Here's how the part is built. I have some questions about the finished solid (model axes, mm). Round coordinates to 2 decimals unless told otherwise and drop trailing zeros. Loops run counter-clockwise (first coordinate to the right, second up) from the corner with the lowest first, then second, coordinate; pieces in that order, holes last. Notation, with made-up numbers: M -11,57.25 L 37,57.25 A8 ccw 37,61.25 Z; hole C -11.5,83 d7. An arc over 180 degrees is marked long. Answer as a JSON object with one key per item and string values.
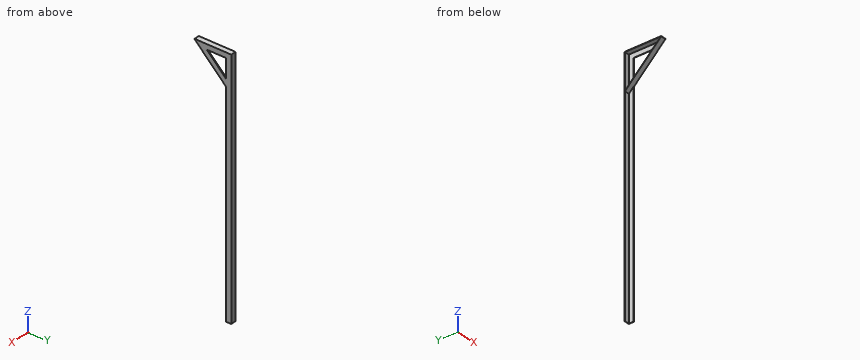
from build123d import *

# Parameters (mm, degrees)
F1_DEPTH  = 2438.4
F2_W      = 3.175
F2_H      = 50.8
F3_DEPTH  = 47.625
F5_DEPTH  = 355.6
F7_DEPTH  = 47.625
F9_DEPTH  = 3.175
F11_DEPTH = 25.4


with BuildPart() as f1:
    # F0 (on Top) → F1 (new body)
    with BuildSketch(Plane.XY):
        Polygon((37.646613, 22.916183), (-13.153387, 22.916183), (-13.153387, 19.741183), (34.471613, 19.741183), (34.471613, -27.883817), (37.646613, -27.883817), align=None)
    extrude(amount=F1_DEPTH)

    # F2 (on face) → F3 (cut)
    with BuildSketch(Plane.XZ.offset(27.883817)):
        with Locations((36.059113, 2413)):
            Rectangle(F2_W, F2_H)
    extrude(amount=-F3_DEPTH, mode=Mode.SUBTRACT)

    # F4 (on face) → F5 (join)
    with BuildSketch(Plane.XZ.offset(-19.741183)):
        Polygon((37.646613, 2438.4), (-13.153387, 2438.4), (-13.153387, 2435.225), (34.471613, 2435.225), (34.471613, 2387.6), (37.646613, 2387.6), align=None)
    extrude(amount=F5_DEPTH)

    # F6 (on face) → F7 (join)
    with BuildSketch(Plane(origin=(34.471613, 0, 0), x_dir=(0, -1, 0), z_dir=(-1, 0, 0))):
        Polygon((-19.741183, 2079.625), (335.858817, 2435.225), (331.368689, 2435.225), (-19.741183, 2084.115128), align=None)
    extrude(amount=F7_DEPTH)

    # F8 (on face) → F9 (join)
    with BuildSketch(Plane.YZ.offset(34.471613)):
        Polygon((-216.391768, 2387.6), (-288.233817, 2387.6), (-27.883817, 2127.25), (-27.883817, 2199.092049), align=None)
    extrude(amount=F9_DEPTH)

    # F10 (on face) → F11 (cut)
    with BuildSketch(Plane(origin=(34.471613, 0, 0), x_dir=(0, -1, 0), z_dir=(-1, 0, 0))):
        Polygon((335.858817, 2387.6), (335.858817, 2435.225), (288.233817, 2387.6), align=None)
    extrude(amount=-F11_DEPTH, mode=Mode.SUBTRACT)


solid = f1.part
Item 1: I want a section at D-D, the plane y = -289.5. Please give me the cut outline in (x, z) (3 decimals), then the cut area to 3 significant figures.
Resolved:
{"outline": "M -13.153,2388.866 L 37.647,2388.866 L 37.647,2438.4 L -13.153,2438.4 L -13.153,2435.225 L 34.472,2435.225 L 34.472,2393.356 L -13.153,2393.356 Z", "area": "522 mm²"}
Item 2: I want a section at A-A, the plane x = 7. Please give me the cut outline in (y, z) (3 decimals), then the cut area to 3 significant figures.
Resolved:
{"outline": "M -335.859,2435.225 L 19.741,2079.625 L 19.741,0 L 22.916,0 L 22.916,2438.4 L -335.859,2438.4 Z; hole M -331.369,2435.225 L 19.741,2084.115 L 19.741,2435.225 Z", "area": "10,500 mm²"}
Item 3: Please list where these lines run through material, in increasing order: probe 1 along Z at (x, y) = (13.5, -121.5) (3 decimals); probe 2 along Z at (x, y) = (16, -203.5) (3 decimals); probe 3 along Y at (x, z) = (31, 1604). Write a range as from..to.
Resolved:
{"probe 1": "2220.866..2225.356, 2435.225..2438.4", "probe 2": "2302.866..2307.356, 2435.225..2438.4", "probe 3": "19.74..22.92"}
Item 4: I want a section at C-C, the plane z = 920. Please give me the cut outline in (x, y).
Resolved:
{"outline": "M -13.15,19.74 L 34.47,19.74 L 34.47,-27.88 L 37.65,-27.88 L 37.65,22.92 L -13.15,22.92 Z"}
Item 5: I'm going to push flat-ended pins straight in: pin 1 Ø12 at (x, z) = (-8, 541.5) entering from -Y; pin 2 Ø12 at (x, y) = (19.5, -25.5) entering from -Z; pin 3 Ø2.5 at (x, z) = (35.5, 2304) entering from -Y. Where does each tip first touch, or does it pass through?
Resolved:
{"pin 1": "y = 19.74", "pin 2": "z = 2118.87", "pin 3": "y = -205.88"}
Item 6: I want a section at B-B, the plane y = -141.5. Please give me the cut outline in (x, z) (3 decimals), then the cut area to 3 significant figures.
Resolved:
{"outline": "M -13.153,2240.866 L 37.647,2240.866 L 37.647,2312.708 L 34.472,2312.708 L 34.472,2245.356 L -13.153,2245.356 Z; M -13.153,2435.225 L 34.472,2435.225 L 34.472,2387.6 L 37.647,2387.6 L 37.647,2438.4 L -13.153,2438.4 Z", "area": "754 mm²"}
